Geometry: see drawing. Coordinates: mm, zero at the bounding-box minimum. A direction names the side the tool comes from. Round coordinates to 2 decimals unless told otherwise and drop trailing zeros. Write each loop counter-clockwise with the first axis right and the second up, starting at its lowest first coordinate (ties: lowest second). Pieces come first, ordered by that corner, then holes. Notation, with made-up numbers: (66.25, 12) - (117.25, 12) arc R29 ccw to (117.25, 39) - close; hole circle Ø7 at (61.25, -3.5). An arc over 180 degrees is marked (long way). One line per item, written item: value. Start each with the question number.
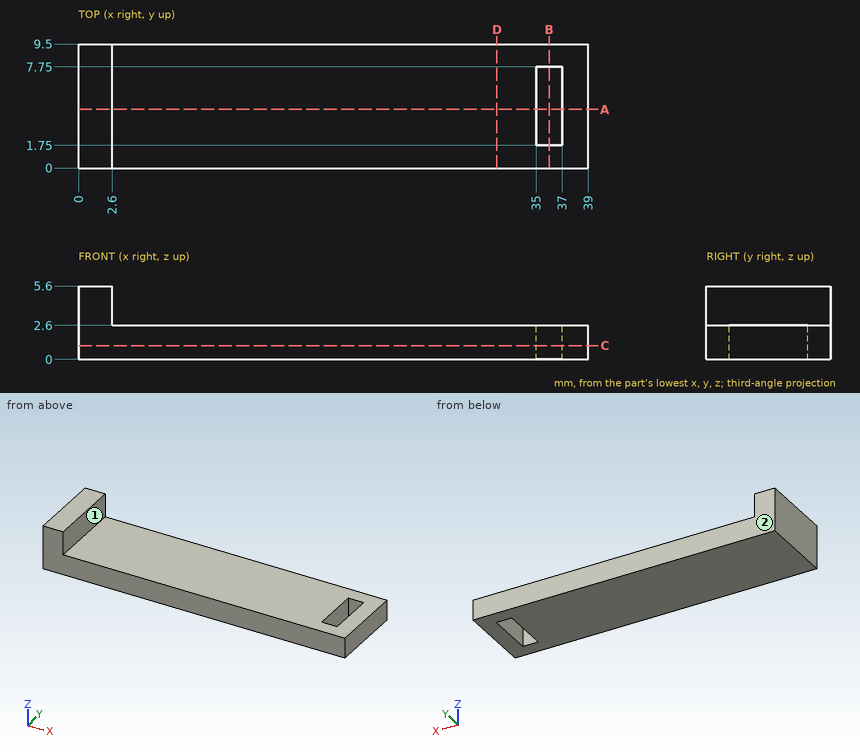
Q1. Material intervals for probe 1 along X at (y, z) = (4, 1.55); probe 2 along Y at (x, z) = (36, 2.1); probe 3 along Z at (x, y) = (21, 7.5), sorted ascending. Write a range as from..to.
Q2. Cut plane D-D, the plane x = 32. Output: boundary loops of the cut face in (y, z), and give its area (3 significant figures).
Q3. Contact query for flat-ended pins moving along their axis: pin 1 Ø2.5 at (y, z) = (5.5, 4.5) entering from +X; pin 2 Ø1.5 at (x, y) = (12, 8) entering from -Z; pin 3 Ø2 at (x, y) = (8, 2.5) entering from +Z. Output: stop coordinate, or through.
Q4. Cut plane C-C, the plane z = 1.05. Output: boundary loops of the cut face in (x, y), and give its area (4 significant figures).
Q5. Access query for the marked faces 1 and 2. Directions: +Z, -Z, +X, -X, +Y, -Y. A direction counts if a zero-diameter tool reaches every point of the face in a straight line with its end or side. Return the directions, or none.
Q6. Cut plane B-B, the plane x = 36. Output: boundary loops of the cut face in (y, z), and give its area (3 significant figures).
Q7. Cut plane A-A, the plane y = 4.5. Output: boundary loops of the cut face in (x, z), and give its area (3 significant figures).
A:
1. probe 1: x = 0..35, 37..39
1. probe 2: y = 0..1.75, 7.75..9.5
1. probe 3: z = 0..2.6
2. outline: (0, 0) - (9.5, 0) - (9.5, 2.6) - (0, 2.6) - close
2. area: 24.7 mm²
3. pin 1: stops at x = 2.6
3. pin 2: stops at z = 0
3. pin 3: stops at z = 2.6
4. outline: (0, 0) - (39, 0) - (39, 9.5) - (0, 9.5) - close; hole (35, 1.75) - (37, 1.75) - (37, 7.75) - (35, 7.75) - close
4. area: 358.5 mm²
5. face 1: +Z, +X, +Y, -Y
5. face 2: +Z, -Z, +X, -X, +Y
6. outline: (0, 0) - (1.75, 0) - (1.75, 2.6) - (0, 2.6) - close; (7.75, 0) - (9.5, 0) - (9.5, 2.6) - (7.75, 2.6) - close
6. area: 9.10 mm²
7. outline: (0, 0) - (35, 0) - (35, 2.6) - (2.6, 2.6) - (2.6, 5.6) - (0, 5.6) - close; (37, 0) - (39, 0) - (39, 2.6) - (37, 2.6) - close
7. area: 104 mm²
